```python
from build123d import *

# Parameters (mm, degrees)
EXTRUDE_THIN1_DEPTH = 20
SKETCH3_R           = 0.75
SKETCH3_W           = 15
SKETCH3_H           = 3
CUT_EXTRUDE1_DEPTH  = 72.214477186


with BuildPart() as part:
    # Sketch2 → Extrude-Thin1 (new body)
    with BuildSketch(Plane(origin=(0, 0, 0), x_dir=(1, 0, 0), z_dir=(0, 1, 0))):
        Polygon((-65.297543233, 13.905764747), (-22.5, 0), (22.5, 0), (65.297543233, 13.905764747), (66.224594216, 11.052595198), (22.975153321, -3), (-22.975153321, -3), (-66.224594216, 11.052595198), align=None)
    extrude(amount=-EXTRUDE_THIN1_DEPTH)

    # Sketch3 → Cut-Extrude1 (cut, through all)
    with BuildSketch(Plane.XY.offset(3)):
        with Locations((-64.799873769, -1)):
            Circle(SKETCH3_R)
        with Locations((-24.399873769, -1)):
            Circle(SKETCH3_R)
        with Locations((-24.399873769, -19)):
            Circle(SKETCH3_R)
        with Locations((-64.799873769, -19)):
            Circle(SKETCH3_R)
        with Locations(Location((64.799873769, -1, 0), (0, 0, 311.57189246))):
            Circle(SKETCH3_R)
        with Locations(Location((24.399873769, -1, 0), (0, 0, 180))):
            Circle(SKETCH3_R)
        with Locations(Location((24.399873769, -19, 0), (0, 0, 180))):
            Circle(SKETCH3_R)
        with Locations(Location((64.799873769, -19, 0), (0, 0, 48.42810754))):
            Circle(SKETCH3_R)
        with Locations((-20.2, -1)):
            Circle(SKETCH3_R)
        with Locations((-20.2, -19)):
            Circle(SKETCH3_R)
        with Locations((20.2, -19)):
            Circle(SKETCH3_R)
        with Locations((20.2, -1)):
            Circle(SKETCH3_R)
        with Locations((0, -1.5)):
            Rectangle(SKETCH3_W, SKETCH3_H)
        with Locations((44.599873769, -1.5)):
            Rectangle(SKETCH3_W, SKETCH3_H)
        with Locations((-44.599873769, -1.5)):
            Rectangle(SKETCH3_W, SKETCH3_H)
    extrude(amount=-CUT_EXTRUDE1_DEPTH, mode=Mode.SUBTRACT)


solid = part.part
```
Input: part model. Units: mm. Frame: model coordinates. A direction names the side the tool comes from. Coordinates: 2 decimals unless noted, no trailing zeros. Loops run counter-clockwise (first coordinate to the right, second up) from the corner with the lowest first, then second, coordinate; pieces in that order, holes last. Notation, with made-up numbers: (6, 79.25) - (43, 79.25) arc R28 ccw to (43, 109.25) - close; hole circle Ø8 at (41, 27). An arc over 180 degrees is marked (long way). Answer in a Markdown table with one row per item.
(1) Cut plane A-A on y = -10.25. Output: boundary loops of the cut face in (x, z).
Model answer:
| item | result |
|---|---|
| outline | (-66.22, -11.05) - (-65.3, -13.91) - (-22.5, 0) - (22.5, 0) - (65.3, -13.91) - (66.22, -11.05) - (22.98, 3) - (-22.98, 3) - close |
(2) Cut plane B-B on z = -12.25. Output: boundary loops of the cut face in (x, y), plus the area to 3 significant figures.
Model answer:
| item | result |
|---|---|
| outline | (-65.84, -20) - (-60.2, -20) - (-60.2, 0) - (-65.84, 0) - close; (60.2, -20) - (65.84, -20) - (65.84, 0) - (60.2, 0) - close; hole circle Ø1.5 at (-64.8, -19); hole circle Ø1.5 at (-64.8, -1); hole circle Ø1.5 at (64.8, -19); hole circle Ø1.5 at (64.8, -1) |
| area | 218 mm² |
(3) Mould query, pull axis X, two halves, no side actions, for faces 1 (the face through (-44.3, -9.86, -3.93)), 2 (the face through (52.1, -2, -8)), 3 (the face through (-22, 0, 1)). Classes: pulls with the +X half, pulls with the -X half, needs draft (parallel to the pull), parting line crosses it, or undercut.
Model answer:
| item | result |
|---|---|
| face 1 | pulls with the -X half |
| face 2 | undercut |
| face 3 | needs draft |
(4) Material intervals for L1, parallel to Y at x = -20.2, z = 1.6; L2, parallel to Z at x = -14, y = -3; L3, parallel to Y at x = 52, z = -9.5, sorted ascending. Write a range as from..to.
Model answer:
| item | result |
|---|---|
| L1 | y = -20..-19.75, -18.25..-1.75, -0.25..0 |
| L2 | z = 0..3 |
| L3 | y = -20..-3 |
(5) Set-up query: faces 4 (the face through (37.1, -2, -3)), 5 (the face through (-37.1, -2, -3)), 6 (the face through (0, -20, 1)), 7 (the face through (0, -10, 0)), 8 (the face through (0, -3, 2)). Return all of +Z, -Z, +X, -X, +Y, -Y with unobstructed straight access to the full face (end or side cutting, diameter ignored); none if empty.
Model answer:
| item | result |
|---|---|
| face 4 | +Z, -Z, +X, +Y |
| face 5 | +Z, -Z, -X, +Y |
| face 6 | +Z, -Z, +X, -X, -Y |
| face 7 | -Z, +Y, -Y |
| face 8 | +Z, -Z, +Y |
(6) Cut plane C-C on x = -39. Output: boundary loops of the cut face in (y, z), plus the area to 3 significant figures.
Model answer:
| item | result |
|---|---|
| outline | (-20, -5.36) - (-3, -5.36) - (-3, -2.21) - (-20, -2.21) - close |
| area | 53.6 mm² |
(7) Pin query (flat end, axial travel): P1, Ø10, axis at x = -5.5, y = -12.5, coming from the -Z side; P2, Ø12, axis at x = -44.5, y = -3.5, coming from the -Z side; P3, Ø3.5, axis at y = -1, z = -3.5, coming from the -X side. Return the tip coordinate at first contact, or that it passes through.
Model answer:
| item | result |
|---|---|
| P1 | stops at z = 0 |
| P2 | stops at z = -9.1 |
| P3 | stops at x = -37.1 |
